The listing builds one solid part. Answer for the finished solid, in the listing's coordinates (mm). A direction names the side the tool comes from. Give positions to 0.01 mm unless a question says otherwise; leave off trailing zeros. Order: outer loops, then holes, each group sorted by start corner. A loop starts at its lowest first (then second) coordinate and runs counter-clockwise, first axis right, second up. Notation, with made-up numbers: (9.25, -36.5) -> (35.25, -36.5) arc R19 ccw to (35.25, -14.5) -> close; hole circle Ø3 at (23, 56.25). An arc over 180 degrees is marked (long way). One line per question, with ' | ' between items. Start each with the question number.
```python
from build123d import *

# Parameters (mm, degrees)
F0_W     = 141.25201
F0_H     = 129.866399
F1_DEPTH = 152.4
F2_W     = 110.178575
F2_H     = 142.77944
F3_DEPTH = 152.4
F4_W     = 100.038202
F4_H     = 138.79922
F5_DEPTH = 152.4


with BuildPart() as f1:
    # F0 (on Top) → F1 (new body)
    with BuildSketch(Plane.XY):
        with Locations((-54.315851, -0.212978)):
            Rectangle(F0_W, F0_H)
    extrude(amount=F1_DEPTH)

    # F2 (on face) → F3 (cut)
    with BuildSketch(Plane.XZ.offset(65.146178)):
        with Locations((-55.089287, 71.38972)):
            Rectangle(F2_W, F2_H)
    extrude(amount=-F3_DEPTH, mode=Mode.SUBTRACT)

    # F4 (on face) → F5 (cut)
    with BuildSketch(Plane.YZ.offset(16.310154)):
        with Locations((-0.600052, 69.39961)):
            Rectangle(F4_W, F4_H)
    extrude(amount=-F5_DEPTH, mode=Mode.SUBTRACT)


solid = f1.part
```
(1) For faces 1 (the face through (-118, 57, 0)), 2 (the face through (8, 49.419, 68)), 3 (the face through (0, 52, 82)), determine the directions among +Z, -Z, +X, -X, +Y, -Y from which every point of the face is accessible in a straight line to the end or side of a thin tool.
(2) Determine the mould class of faces 4 (the face through (16.31, -1, 144)), 5 (the face through (-117, -50.619, 68)), 6 (the face through (-110.179, 52, 82)) for opening direction X: pulls with the +X half, pulls with the -X half, needs draft (parallel to the pull), parting line crosses it, or undercut.
(3) The part is cut by section C-C on y = 8. Determine the outline of the cut face in (x, z), plus the area to 3 significant figures.
(4) The part is cut by section B-B on x = -114.5. Determine the outline of the cut face in (y, z), plus the area to 3 significant figures.
(5) Given P1, Ø1, axis at x = -40.5, y = 34, coming from the -Z side; P2, Ø7.5, axis at x = -116.5, y = 5, coming from the -Z side; P3, Ø10, axis at x = -7.5, z = 122, coming from the -Y side, each flat-ended and moving along its own axis, determine where each tip first touches the part or whether it passes through.
(6) Consider line 1 (Y direction, x = 3.5, z = 55.5); line 2 (Z direction, x = -5, y = -22); line 3 (X direction, y = 51, z = 46.5). Determine where each line is inside the solid, lowest interval first.
(7) The part is cut by section A-A on z = 119.5. Determine the outline of the cut face in (x, y).
(8) The part is cut by section D-D on x = -93.5. Determine the outline of the cut face in (y, z), plus the area to 3 significant figures.
Result sheet:
1) face 1: -Z, +X, -X, +Y, -Y | face 2: -Z, +X, -X | face 3: -Z, +Y, -Y
2) face 4: pulls with the +X half | face 5: needs draft | face 6: undercut
3) outline: (-124.94, 138.8) -> (-110.18, 138.8) -> (-110.18, 142.78) -> (0, 142.78) -> (0, 138.8) -> (16.31, 138.8) -> (16.31, 152.4) -> (-124.94, 152.4) -> close | area: 1,480 mm^2
4) outline: (-65.15, 0) -> (-50.62, 0) -> (-50.62, 138.8) -> (49.42, 138.8) -> (49.42, 0) -> (64.72, 0) -> (64.72, 152.4) -> (-65.15, 152.4) -> close | area: 5,910 mm^2
5) P1: stops at z = 142.78 | P2: stops at z = 138.8 | P3: passes through
6) line 1: y = -65.15 to -50.62, 49.42 to 64.72 | line 2: z = 142.78 to 152.4 | line 3: x = -124.94 to -110.18, 0 to 16.31
7) outline: (-124.94, -65.15) -> (-110.18, -65.15) -> (-110.18, -50.62) -> (-124.94, -50.62) -> close; (-124.94, 49.42) -> (-110.18, 49.42) -> (-110.18, 64.72) -> (-124.94, 64.72) -> close; (0, -65.15) -> (16.31, -65.15) -> (16.31, -50.62) -> (0, -50.62) -> close; (0, 49.42) -> (16.31, 49.42) -> (16.31, 64.72) -> (0, 64.72) -> close
8) outline: (-65.15, 142.78) -> (64.72, 142.78) -> (64.72, 152.4) -> (-65.15, 152.4) -> close | area: 1,250 mm^2
